Could you check a few things on this model? Use its own coordinates, in mm. A direction names the side the tool comes from. Give positions to 0.01 mm unless a question says otherwise; leave off trailing zeros. Loops run counter-clockwise (first coordinate to the right, second up) from the corner with the lowest first, then second, coordinate; pieces in that order, holes last. Notation, with made-up numbers: M 78,18.5 L 115,18.5 A21 cw 115,37.5 Z; hole C 82,-2 d7. An arc over 180 degrees is marked long. Use a Markdown table: item, result. Add a question column.
1) We'd pull the mould along X, two halves only. Please class faces 1 (the flat face through (2, 0, -50.8)), 2 (the cylindrical face through (-215.888, -0.133, 1.117)), 3 (the conical face through (-203.985, 6.335, 0.855)): +X half, -X half, draft (parallel to the pull), parting line (faces both ways), or undercut.
2) Which directions (+Z, -Z, +X, -X, +Y, -Y) give clear straight access to the entire face, cutting with the end or side of a thin tool? Please do faces 4 (the flat face through (-2.31, 7.8, 44.36)), 5 (the cylindrical face through (215.888, -0.133, -1.117)), 6 (the flat face through (-2, 0, 50.8)), 7 (the flat face through (-2.311, -7.847, 44.539)), 8 (the cylindrical face through (-203.19, 0.09, 0.84)).
3) If I drill on line 1 along Z through (x, y) = (-34.5, -3.25); line 2 along X through (y, z) = (-2.5, 16.5); line 3 along Z through (x, y) = (185.5, -3), over which ranges is the centre line in solid material (lowest first)? Write a range as [from, to].
4) Suppose I cut it at C-C on z = 0. List the corners of the cut face in (x, y) for me (3 decimals).
5) Suppose I cut it at B-B on x = 52.5. List the corners of the cut face in (y, z) for me (3 decimals), and give its area (3 significant figures).
6) Suppose I cut it at A-A on y = 0.5. List the corners of the cut face in (x, z) for me.
7) Will these pins go through, and if not, where does the flat tip stop? pin 1 Ø4 at (y, z) = (-2, -40) entering from -X; pin 2 Ø3 at (y, z) = (-1.5, 26) entering from +X; pin 3 Ø5 at (y, z) = (2, 33.5) entering from -X.
```python
from build123d import *


with BuildPart() as part:
    # Sweep1: sweep along a path in Sketch1
    with BuildLine(Plane(origin=(0, 0, 0), x_dir=(1, 0, 0), z_dir=(0, 1, 0))) as sweep1_path:
        Line((165.1, -50.8), (-165.1, -50.8))
        ThreePointArc((-165.1, -50.8), (-215.9, 0), (-165.1, 50.8))
        Line((-165.1, 50.8), (165.1, 50.8))
        ThreePointArc((165.1, 50.8), (215.9, 0), (165.1, -50.8))
    # Sketch2 → Sweep1 (sweep)
    with BuildSketch(Plane(origin=(-165.1, 0, -50.8), x_dir=(0, 0, 1), z_dir=(-1, 0, 0))):
        Polygon((0, 0), (0, 9.525), (12.7, 6.122045256), (12.7, -6.122045256), (0, -9.525), align=None)
    sweep(path=sweep1_path.line)


solid = part.part
```
Answer block:
| question | item | result |
|---|---|---|
| 1 | face 1 | draft |
| 1 | face 2 | -X half |
| 1 | face 3 | undercut |
| 2 | face 4 | +Y |
| 2 | face 5 | +X, +Y, -Y |
| 2 | face 6 | +Z, +X, -X, +Y, -Y |
| 2 | face 7 | -Y |
| 2 | face 8 | +Y, -Y |
| 3 | line 1 | z = [-50.8, -38.1], [38.1, 50.8] |
| 3 | line 2 | x = [-213.15, -199.44], [199.44, 213.15] |
| 3 | line 3 | z = [-46.52, -32.18], [32.18, 46.52] |
| 4 | outline | M -215.9,-9.525 L -203.2,-6.122 L -203.2,6.122 L -215.9,9.525 Z; M 203.2,-6.122 L 215.9,-9.525 L 215.9,9.525 L 203.2,6.122 Z |
| 5 | outline | M -9.525,-50.8 L 9.525,-50.8 L 6.122,-38.1 L -6.122,-38.1 Z; M -9.525,50.8 L -6.122,38.1 L 6.122,38.1 L 9.525,50.8 Z |
| 5 | area | 397 mm^2 |
| 6 | outline | M -165.1,-50.8 L 165.1,-50.8 A50.8 ccw 165.1,50.8 L -165.1,50.8 A50.8 ccw Z; hole M -165.1,-38.1 L 165.1,-38.1 A38.1 ccw 165.1,38.1 L -165.1,38.1 A38.1 ccw Z |
| 7 | pin 1 | stops at x = -198.81 |
| 7 | pin 2 | stops at x = 209.6 |
| 7 | pin 3 | stops at x = -205.34 |
